Verification items for the finished model (mm, model axes). A direction names the side the tool comes from. Round coordinates to 2 decimals unless told otherwise and drop trailing zeros. Loops run counter-clockwise (first coordinate to the right, second up) from the corner with the lowest first, then second, coordinate; pieces in that order, holes last. Notation, with made-up numbers: (43, 12.25) - (73, 12.25) arc R12 cw to (73, 29.25) - close; hole circle Ø8 at (79, 6). An arc over 180 degrees is marked (long way). Use CSV: the item, a comma, the result in double quotes.
```python
from build123d import *

# Parameters (mm, degrees)
CORTE_W                 = 6.05
CORTE_H                 = 6
SALIENTE_EXTRUIR1_DEPTH = 6


with BuildPart() as part:
    # Corte → Saliente-Extruir1 (new body)
    with BuildSketch(Plane.XY):
        with BuildLine():
            Line((113.357081542, 26.21056425), (157.224997542, 51.53767625))
            add(Edge.make_bspline(
                [(157.224997542, 51.53767625), (159.190322542, 52.67288025), (160.400350542, 54.76749825), (160.399997542, 57.03698825)],
                knots=[0, 0, 0, 0, 1, 1, 1, 1], degree=3))
            Line((160.399997542, 57.03698825), (160.399997542, 142.96314225))
            add(Edge.make_bspline(
                [(160.399997542, 142.96314225), (160.399645542, 145.23256125), (159.190675542, 147.32841425), (157.224997542, 148.46259425)],
                knots=[0, 0, 0, 0, 1, 1, 1, 1], degree=3))
            Line((157.224997542, 148.46259425), (113.357081542, 173.78956925))
            add(Edge.make_bspline(
                [(113.357081542, 173.78956925), (111.391403542, 174.92375025), (108.972053542, 174.92480825), (107.007081542, 173.78956925)],
                knots=[0, 0, 0, 0, 1, 1, 1, 1], degree=3))
            Line((107.007081542, 173.78956925), (32.592792542, 130.82652825))
            add(Edge.make_bspline(
                [(32.592792542, 130.82652825), (30.627711542, 129.69128925), (29.417379542, 127.59649425), (29.417792542, 125.32707525)],
                knots=[0, 0, 0, 0, 1, 1, 1, 1], degree=3))
            Line((29.417792542, 125.32707525), (29.417792542, 74.67277225))
            add(Edge.make_bspline(
                [(29.417792542, 74.67277225), (29.418206542, 72.40335325), (30.627157542, 70.30785325), (32.592792542, 69.17367225)],
                knots=[0, 0, 0, 0, 1, 1, 1, 1], degree=3))
            Line((32.592792542, 69.17367225), (107.007081542, 26.21056425))
            add(Edge.make_bspline(
                [(107.007081542, 26.21056425), (108.972758542, 25.07630125), (111.391756542, 25.07533725), (113.357081542, 26.21056425)],
                knots=[0, 0, 0, 0, 1, 1, 1, 1], degree=3))
        make_face()
        Polygon((82.209667177, 45.146306921), (87.405777131, 42.146233364), (90.430851301, 47.385644235), (85.234741347, 50.385717791), align=None, mode=Mode.SUBTRACT)
        Polygon((59.219111627, 65.405686508), (64.415251823, 62.405665331), (61.39023047, 57.166223967), (56.194090274, 60.166245143), align=None, mode=Mode.SUBTRACT)
        Polygon((115.970526872, 32.338235445), (121.166681404, 35.338231793), (118.141685086, 40.577687612), (112.945530555, 37.577691264), align=None, mode=Mode.SUBTRACT)
        Polygon((147.586560764, 57.577666916), (150.611557081, 52.338211097), (145.41540255, 49.338214749), (142.390406233, 54.577670568), align=None, mode=Mode.SUBTRACT)
        Polygon((59.219036883, 134.594225381), (64.415170597, 137.594257784), (61.390137924, 142.833692613), (56.194004209, 139.83366021), align=None, mode=Mode.SUBTRACT)
        Polygon((82.20954866, 154.853654641), (87.405652132, 157.853739425), (90.430737623, 152.61433509), (85.234634151, 149.614250307), align=None, mode=Mode.SUBTRACT)
        Polygon((112.945395686, 162.422336706), (115.970380683, 167.661799061), (121.166541696, 164.66181394), (118.141556699, 159.422351585), align=None, mode=Mode.SUBTRACT)
        Polygon((147.586469106, 142.422435899), (150.611454103, 147.661898254), (145.41529309, 150.661883375), (142.390308093, 145.42242102), align=None, mode=Mode.SUBTRACT)
        with Locations((153.374997542, 83.000060929)):
            Rectangle(CORTE_W, CORTE_H, mode=Mode.SUBTRACT)
        Polygon((150.349997542, 120.000060929), (156.399997542, 120.000060929), (156.399997542, 114.000060929), (150.349997542, 114.000054393), align=None, mode=Mode.SUBTRACT)
        with BuildLine():
            add(Edge.make_bspline(
                [(51.13479556, 75.869945702), (51.134797227, 75.098420702), (50.509323579, 74.47294435), (49.737798579, 74.472942683)],
                knots=[0, 0, 0, 0, 1, 1, 1, 1], degree=3))
            add(Edge.make_bspline(
                [(49.737798579, 74.472942683), (48.966273579, 74.472941016), (48.340797227, 75.098414665), (48.34079556, 75.869939665)],
                knots=[0, 0, 0, 0, 1, 1, 1, 1], degree=3))
            add(Edge.make_bspline(
                [(48.34079556, 75.869939665), (48.340793893, 76.641464665), (48.966267542, 77.266941016), (49.737792542, 77.266942683)],
                knots=[0, 0, 0, 0, 1, 1, 1, 1], degree=3))
            add(Edge.make_bspline(
                [(49.737792542, 77.266942683), (50.509317542, 77.26694435), (51.134793893, 76.641470702), (51.13479556, 75.869945702)],
                knots=[0, 0, 0, 0, 1, 1, 1, 1], degree=3))
        make_face(mode=Mode.SUBTRACT)
        with BuildLine():
            add(Edge.make_bspline(
                [(52.40444356, 124.12993061), (52.404445227, 123.35840561), (51.778971579, 122.732929259), (51.007798579, 122.732927592)],
                knots=[0, 0, 0, 0, 1, 1, 1, 1], degree=3))
            add(Edge.make_bspline(
                [(51.007798579, 122.732927592), (50.235921579, 122.732925925), (49.610445227, 123.358399573), (49.61044356, 124.129924573)],
                knots=[0, 0, 0, 0, 1, 1, 1, 1], degree=3))
            add(Edge.make_bspline(
                [(49.61044356, 124.129924573), (49.610441893, 124.901449573), (50.235915542, 125.526925925), (51.007792542, 125.526927592)],
                knots=[0, 0, 0, 0, 1, 1, 1, 1], degree=3))
            add(Edge.make_bspline(
                [(51.007792542, 125.526927592), (51.778965542, 125.526929259), (52.404441893, 124.90145561), (52.40444356, 124.12993061)],
                knots=[0, 0, 0, 0, 1, 1, 1, 1], degree=3))
        make_face(mode=Mode.SUBTRACT)
        with BuildLine():
            add(Edge.make_bspline(
                [(103.20479556, 108.88993061), (103.204797227, 108.11840561), (102.579323579, 107.492929259), (101.807798579, 107.492927592)],
                knots=[0, 0, 0, 0, 1, 1, 1, 1], degree=3))
            add(Edge.make_bspline(
                [(101.807798579, 107.492927592), (101.036273579, 107.492925925), (100.410797227, 108.118399573), (100.41079556, 108.889924573)],
                knots=[0, 0, 0, 0, 1, 1, 1, 1], degree=3))
            add(Edge.make_bspline(
                [(100.41079556, 108.889924573), (100.410793893, 109.661449573), (101.036267542, 110.286925925), (101.807792542, 110.286927592)],
                knots=[0, 0, 0, 0, 1, 1, 1, 1], degree=3))
            add(Edge.make_bspline(
                [(101.807792542, 110.286927592), (102.579317542, 110.286929259), (103.204793893, 109.66145561), (103.20479556, 108.88993061)],
                knots=[0, 0, 0, 0, 1, 1, 1, 1], degree=3))
        make_face(mode=Mode.SUBTRACT)
        with BuildLine():
            add(Edge.make_bspline(
                [(103.20479556, 80.94993061), (103.204797227, 80.17840561), (102.579323579, 79.552929259), (101.807798579, 79.552927592)],
                knots=[0, 0, 0, 0, 1, 1, 1, 1], degree=3))
            add(Edge.make_bspline(
                [(101.807798579, 79.552927592), (101.036273579, 79.552925925), (100.410797227, 80.178399573), (100.41079556, 80.949924573)],
                knots=[0, 0, 0, 0, 1, 1, 1, 1], degree=3))
            add(Edge.make_bspline(
                [(100.41079556, 80.949924573), (100.410793893, 81.721449573), (101.036267542, 82.346925925), (101.807792542, 82.346927592)],
                knots=[0, 0, 0, 0, 1, 1, 1, 1], degree=3))
            add(Edge.make_bspline(
                [(101.807792542, 82.346927592), (102.579317542, 82.346929259), (103.204793893, 81.72145561), (103.20479556, 80.94993061)],
                knots=[0, 0, 0, 0, 1, 1, 1, 1], degree=3))
        make_face(mode=Mode.SUBTRACT)
        with BuildLine():
            add(Edge.make_bspline(
                [(133.68479556, 75.86993061), (133.684797227, 75.09840561), (133.059323579, 74.472929259), (132.287798579, 74.472927592)],
                knots=[0, 0, 0, 0, 1, 1, 1, 1], degree=3))
            add(Edge.make_bspline(
                [(132.287798579, 74.472927592), (131.516273579, 74.472925925), (130.890797227, 75.098399573), (130.89079556, 75.869924573)],
                knots=[0, 0, 0, 0, 1, 1, 1, 1], degree=3))
            add(Edge.make_bspline(
                [(130.89079556, 75.869924573), (130.890793893, 76.641449573), (131.516267542, 77.266925925), (132.287792542, 77.266927592)],
                knots=[0, 0, 0, 0, 1, 1, 1, 1], degree=3))
            add(Edge.make_bspline(
                [(132.287792542, 77.266927592), (133.059317542, 77.266929259), (133.684793893, 76.64145561), (133.68479556, 75.86993061)],
                knots=[0, 0, 0, 0, 1, 1, 1, 1], degree=3))
        make_face(mode=Mode.SUBTRACT)
        with BuildLine():
            add(Edge.make_bspline(
                [(127.33479556, 124.12993061), (127.334797227, 123.35840561), (126.709323579, 122.732929259), (125.937798579, 122.732927592)],
                knots=[0, 0, 0, 0, 1, 1, 1, 1], degree=3))
            add(Edge.make_bspline(
                [(125.937798579, 122.732927592), (125.166273579, 122.732925925), (124.540797227, 123.358399573), (124.54079556, 124.129924573)],
                knots=[0, 0, 0, 0, 1, 1, 1, 1], degree=3))
            add(Edge.make_bspline(
                [(124.54079556, 124.129924573), (124.540793893, 124.901449573), (125.166267542, 125.526925925), (125.937792542, 125.526927592)],
                knots=[0, 0, 0, 0, 1, 1, 1, 1], degree=3))
            add(Edge.make_bspline(
                [(125.937792542, 125.526927592), (126.709317542, 125.526929259), (127.334793893, 124.90145561), (127.33479556, 124.12993061)],
                knots=[0, 0, 0, 0, 1, 1, 1, 1], degree=3))
        make_face(mode=Mode.SUBTRACT)
    extrude(amount=-SALIENTE_EXTRUIR1_DEPTH)


solid = part.part
```
1) Cross-section at B-B, the plane x = 42. Record the cut outline in (y, z), then the cut area to 3 significant figures.
Returned:
outline,"(63.74, -6) - (136.26, -6) - (136.26, 0) - (63.74, 0) - close"
area,"435 mm²"
2) Cross-section at A-A, the plane z = -2.25. Count the separate pieces of the cut face and the enclosed holes in it, then the cut area to 3 significant figures.
Returned:
separate pieces,"1"
enclosed holes,"16"
area,"14,200 mm²"
3) Access from +Z, -Z, +X, -X, +Y, -Y to the whole of each face (thin tool, end or side, straight path). Record for faces 1 (the face through (83.74, 47.8, -2.96)), 2 (the face through (135.6, 160.95, -2.96)).
Returned:
face 1,"+Z, -Z"
face 2,"+Z, -Z, +X, +Y"
4) Cross-section at C-C, the plane x = 97.5. Record the cut outline in (y, z).
Returned:
outline,"(31.7, -6) - (168.3, -6) - (168.3, 0) - (31.7, 0) - close"
5) Gauge pin test, flat ends, axial feed: pin 1 Ø3 at (x, z) = (154, -4.5) entering from +Y; pin 2 Ø8 at (x, y) = (122, 153) entering from +Z; pin 3 Ø1.8 at (x, z) = (153.5, -3.5) entering from -Y. Record the tip position at first contact, or that the pin passes through.
Returned:
pin 1,"stops at y = 151.19"
pin 2,"stops at z = 0"
pin 3,"stops at y = 48.87"
6) Mould release check, pull along X, two halves, no side actions. Record for faces 3 (the face through (94, 101, -6)), 4 (the face through (88.897, 44.729, -2.958)), 5 (the face through (134.984, 38.697, -2.958)): +X half, -X half, draft (parallel to the pull), parting line (faces both ways), or undercut.
Returned:
face 3,"draft"
face 4,"undercut"
face 5,"+X half"
7) Thickness scan on probe 1 along Y at (x, z) = (102, -3.25); probe 2 along Y at (x, z) = (116.5, -1); probe 3 along X at (y, z) = (142, -5). Record the ranges inside material, lowest first. Write a range as [from, to].
Returned:
probe 1,"y = [29.1, 79.57], [82.33, 107.51], [110.27, 170.9]"
probe 2,"y = [28.03, 32.64], [39.63, 160.37], [167.36, 171.98]"
probe 3,"x = [51.95, 59.95], [61.87, 160.4]"
